Geometry: final body of the model. Coordinates: model frame, mm. A direction names the side the tool comes from. Give positions to 0.01 mm unless a question says otherwise; leave off trailing zeros. Loops run counter-clockwise (first coordinate to the right, second up) from the corner with the lowest first, then second, coordinate; pieces in that order, holes last. Notation, with made-up numbers: (50, 51) -> (66, 51) arc R27 ccw to (66, 86) -> close; hole circle Ø2 at (76, 47.5). An arc over 180 degrees is marked (long way). Answer in a Markdown table with one row per item. Add a question column.
1) Section query C-C (x = -7.75). Return the cut outline in (y, z).
2) Section query A-A (y = 21). Return the cut outline in (x, z).
3) First-contact query: P1, Ø5, axis at x = 15.5, y = 7, coming from the -Z side; P2, Ø1, axis at x = -9, y = 20.5, coming from the +Z side; P3, Ø1.5, axis at x = -16, z = 7, coming from the +Y side. Flat tips, straight axial feed; report the tip coordinate or a pass-through.
4) Draft query along Y for faces 5 (the cylindrical face through (-8.856, -5.41, 8.465)), 6 (the conical face through (16.2, 18.88, 7.08)), 7 (the cylindrical face through (-15.73, 23.44, 8.22)). Return one class per face: +Y half, -Y half, draft (parallel to the pull), parting line (faces both ways), or undercut.
5) Line query: line 1 (Y direction, x = -7.75, z = 13.9); line 2 (X direction, y = 7, z = 7.75); line 3 (X direction, y = -19.5, z = 10). Output: solid intervals per line, ascending. Write a range as from..to.
6) Access query for faces 1 (the cylindrical face through (6.644, -5.41, 8.465)), 2 (the cylindrical face through (8.75, -22.43, 6.95)), 3 (the flat face through (6, 20, 11)), 4 (the cylindrical face through (-17.43, -24.9, 6.08)). Directions: +Z, -Z, +X, -X, +Y, -Y. A direction counts if a zero-diameter tool reaches every point of the face in a straight line with its end or side. Return the directions, or none.
7) Section query B-B (x = 0). Return the cut outline in (y, z), plus the area to 3 significant figures.
8) Section query D-D (z = 3.5). Give the number of separate pieces and of enclosed holes in the cut face, plus the area to 3 significant figures.
```python
from build123d import *

# Parameters (mm, degrees)
SKETCH1_W             = 40
SKETCH1_H             = 55
SKETCH1_R             = 6
SKETCH1_R_2           = 1.5
BOSS_EXTRUDE1_DEPTH   = 15
SKETCH2_R             = 18.5
CUT_EXTRUDE1_DEPTH    = 6
M3_TAPPED_HOLE1_D     = 2.5
M3_TAPPED_HOLE1_DEPTH = 10
M3_TAPPED_HOLE1_TIP   = 0.751075774
M3_TAPPED_HOLE2_D     = 2.5
M3_TAPPED_HOLE2_DEPTH = 8
M3_TAPPED_HOLE2_TIP   = 0.751075774
SKETCH7_R             = 3.25
CUT_EXTRUDE2_DEPTH    = 4
CUT_EXTRUDE3_DEPTH    = 12
FILLET1_R             = 2
SKETCH10_W            = 3
SKETCH10_H            = 48
BOSS_EXTRUDE2_DEPTH   = 15


with BuildPart() as part:
    # Sketch1 → Boss-Extrude1 (new body)
    with BuildSketch(Plane.XY):
        Rectangle(SKETCH1_W, SKETCH1_H)
        Circle(SKETCH1_R, mode=Mode.SUBTRACT)
        with Locations((15.5, 7)):
            Circle(SKETCH1_R_2, mode=Mode.SUBTRACT)
        with Locations((7.75, -6.423393759)):
            Circle(SKETCH1_R_2, mode=Mode.SUBTRACT)
        with Locations((-7.75, -6.423393759)):
            Circle(SKETCH1_R_2, mode=Mode.SUBTRACT)
        with Locations((-15.5, 7)):
            Circle(SKETCH1_R_2, mode=Mode.SUBTRACT)
        with Locations((-7.75, 20.423393759)):
            Circle(SKETCH1_R_2, mode=Mode.SUBTRACT)
        with Locations((7.75, 20.423393759)):
            Circle(SKETCH1_R_2, mode=Mode.SUBTRACT)
    extrude(amount=BOSS_EXTRUDE1_DEPTH)

    # Sketch2 → Cut-Extrude1 (cut)
    with BuildSketch(Plane(origin=(0, 0, 0), x_dir=(-1, 0, 0), z_dir=(0, 0, -1))):
        with Locations((0, 7)):
            Circle(SKETCH2_R)
    extrude(amount=-CUT_EXTRUDE1_DEPTH, mode=Mode.SUBTRACT)

    # M3 Tapped Hole1
    with Locations(Plane(origin=(0, -27.5, 0), x_dir=(-1, 0, 0), z_dir=(0, -1, 0))):
        with Locations((-10, -7), (10, -7)):
            Hole(M3_TAPPED_HOLE1_D / 2, depth=M3_TAPPED_HOLE1_DEPTH)
            with Locations((0, 0, -(M3_TAPPED_HOLE1_DEPTH + M3_TAPPED_HOLE1_TIP / 2))):  # 118° drill point
                Cone(0, M3_TAPPED_HOLE1_D / 2, M3_TAPPED_HOLE1_TIP, mode=Mode.SUBTRACT)

    # M3 Tapped Hole2
    with Locations(Plane(origin=(0, 27.5, 0), x_dir=(1, 0, 0), z_dir=(0, 1, 0))):
        with Locations((-16, -7), (16, -7)):
            Hole(M3_TAPPED_HOLE2_D / 2, depth=M3_TAPPED_HOLE2_DEPTH)
            with Locations((0, 0, -(M3_TAPPED_HOLE2_DEPTH + M3_TAPPED_HOLE2_TIP / 2))):  # 118° drill point
                Cone(0, M3_TAPPED_HOLE2_D / 2, M3_TAPPED_HOLE2_TIP, mode=Mode.SUBTRACT)

    # Sketch7 → Cut-Extrude2 (cut)
    with BuildSketch(Plane.XY.offset(15)):
        with Locations((-7.75, 20.423393759)):
            Circle(SKETCH7_R)
        with Locations((7.75, 20.423393759)):
            Circle(SKETCH7_R)
        with Locations((15.5, 7)):
            Circle(SKETCH7_R)
        with Locations((7.75, -6.423393759)):
            Circle(SKETCH7_R)
        with Locations((-7.75, -6.423393759)):
            Circle(SKETCH7_R)
        with Locations((-15.5, 7)):
            Circle(SKETCH7_R)
    extrude(amount=-CUT_EXTRUDE2_DEPTH, mode=Mode.SUBTRACT)

    # Sketch9 → Cut-Extrude3 (cut)
    with BuildSketch(Plane(origin=(0, 0, 0), x_dir=(-1, 0, 0), z_dir=(0, 0, -1))):
        with BuildLine():
            Line((-18, -25.5), (-13.25, -25.5))
            Line((-13.25, -25.5), (-13.25, -15.5))
            Line((-13.25, -15.5), (-6.75, -15.5))
            Line((-6.75, -15.5), (-6.75, -25.5))
            Line((-6.75, -25.5), (6.75, -25.5))
            Line((6.75, -25.5), (6.75, -15.5))
            Line((6.75, -15.5), (13.25, -15.5))
            Line((13.25, -15.5), (13.25, -25.5))
            Line((13.25, -25.5), (18, -25.5))
            Line((18, -25.5), (18, -2.810708435))
            ThreePointArc((18, -2.810708435), (0, -13.5), (-18, -2.810708435))
            Line((-18, -2.810708435), (-18, -25.5))
        make_face()
    extrude(amount=-CUT_EXTRUDE3_DEPTH, mode=Mode.SUBTRACT)

    # Fillet1
    fillet1_edges = [part.edges().sort_by_distance(p)[0] for p in [
        (18, -25.5, 6),
        (18, -2.810708435, 6),
        (-18, -2.810708435, 6),
        (-18, -25.5, 6),
        (-13.25, -25.5, 6),
        (-13.25, -15.5, 6),
        (-6.75, -15.5, 6),
        (-6.75, -25.5, 6),
        (6.75, -25.5, 6),
        (6.75, -15.5, 6),
        (13.25, -15.5, 6),
        (13.25, -25.5, 6),
    ]]
    fillet(fillet1_edges, radius=FILLET1_R)

    # Sketch10 → Boss-Extrude2 (add)
    with BuildSketch(Plane.XY.offset(15)):
        with Locations((-21.5, 3.5)):
            Rectangle(SKETCH10_W, SKETCH10_H)
        with Locations((21.5, 3.5)):
            Rectangle(SKETCH10_W, SKETCH10_H)
    extrude(amount=BOSS_EXTRUDE2_DEPTH)


with BuildPart() as boss_extrude2_kept_piece:
    # of the separate pieces the step leaves, the one the design keeps (boss_extrude2_pieces_kept)
    add(part.part.solids().sort_by_distance((18, -8.81929202, 0))[0])


solid = boss_extrude2_kept_piece.part
```
Evaluation:
| question | item | result |
|---|---|---|
| 1 | outline | (-27.5, 0) -> (-15.77, 0) -> (-15.77, 12) -> (-11.98, 12) -> (-11.98, 0) -> (-9.8, 0) -> (-9.8, 6) -> (-7.92, 6) -> (-7.92, 11) -> (-9.67, 11) -> (-9.67, 15) -> (-27.5, 15) -> close; (-4.92, 6) -> (18.92, 6) -> (18.92, 11) -> (17.17, 11) -> (17.17, 15) -> (-3.17, 15) -> (-3.17, 11) -> (-4.92, 11) -> close; (21.92, 6) -> (23.8, 6) -> (23.8, 0) -> (27.5, 0) -> (27.5, 15) -> (23.67, 15) -> (23.67, 11) -> (21.92, 11) -> close |
| 2 | outline | (-20, 0) -> (-12.09, 0) -> (-12.09, 6) -> (-9.13, 6) -> (-9.13, 11) -> (-10.95, 11) -> (-10.95, 15) -> (-20, 15) -> close; (-6.37, 6) -> (6.37, 6) -> (6.37, 11) -> (4.55, 11) -> (4.55, 15) -> (-4.55, 15) -> (-4.55, 11) -> (-6.37, 11) -> close; (9.13, 6) -> (12.09, 6) -> (12.09, 0) -> (20, 0) -> (20, 15) -> (10.95, 15) -> (10.95, 11) -> (9.13, 11) -> close; hole circle Ø2.5 at (-16, 7); hole circle Ø2.5 at (16, 7) |
| 3 | P1 | z = 6 |
| 3 | P2 | z = 11 |
| 3 | P3 | y = 19.2 |
| 4 | face 5 | undercut |
| 4 | face 6 | +Y half |
| 4 | face 7 | draft |
| 5 | line 1 | -27.5..-9.67, -3.17..17.17, 23.67..27.5 |
| 5 | line 2 | -20..-17, -14..14, 17..20 |
| 5 | line 3 | -20..-18, -13.25..-6.75, 6.75..13.25, 18..20 |
| 6 | face 1 | +Z, -Z |
| 6 | face 2 | -Y |
| 6 | face 3 | +Z |
| 6 | face 4 | -Z |
| 7 | outline | (-27.5, 0) -> (-25.5, 0) -> (-25.5, 12) -> (-13.5, 12) -> (-13.5, 0) -> (-11.5, 0) -> (-11.5, 6) -> (-6, 6) -> (-6, 15) -> (-27.5, 15) -> close; (6, 6) -> (25.5, 6) -> (25.5, 0) -> (27.5, 0) -> (27.5, 15) -> (6, 15) -> close |
| 7 | area | 351 mm² |
| 8 | separate pieces | 1 |
| 8 | enclosed holes | 2 |
| 8 | area | 726 mm² |
